Model file for the job. Use its own axes, mm. Face numbers are marked on the shaded views. A direction names the side the tool comes from. Coordinates: 2 decimals unless noted, no trailing zeros. Write each loop counter-clockwise with the first axis right and the second up, starting at its lowest first coordinate (ties: lowest second). Pieces come first, ordered by that corner, then holes. Notation, with made-up numbers: M -22,67 L -3,67 A21 ccw -3,85 Z; hole C 22,7 d4. An arc over 180 degrees is marked long. Put each result on its own line as item: value. Start each with the question number.
Q1. Drop flat-ended pins along their axis: pin 1 (4.5 mm diameter, centred on x = 13.5, y = -1.5, fed in from -Z); pin 2 (0.8 mm diameter, centred on y = -2.5, z = 1.5, fed in from +X). Give the stop position or say it passes through.
Q2. Cut at A-A (x = 17.75). Write the cut outline in (y, z), then the cut area to 3 significant figures.
Q3. Which spindle directions (+Z, -Z, +X, -X, +Y, -Y) get a long thin tool onto all of the face, cutting with end or side? Do the marked faces 1 and 2. Say none if no direction does.
Q4. Cut at C-C (z = 5.75). Write the cut outline in (x, y), then the cut area to 3 significant figures.
Q5. Pull direction X, two halves, no side cores. Call the marked faces 3, 4 and 5: pulls with the +X half, pulls with the -X half, needs draft (parallel to the pull), parting line crosses it, or undercut.
Q6. Cut at D-D (x = 14.25). Write the cut outline in (y, z).
Q7. Cut at B-B (y = 3.25). Write the cut outline in (x, z).
Q8. Drill centre lines: line 1 along Y through (x, z) = (26, 7.5); line 2 along X through (y, z) = (-1.25, 1.25); line 3 along X through (y, z) = (-4.5, 9.75). Where is each one in solid material? Low to high.
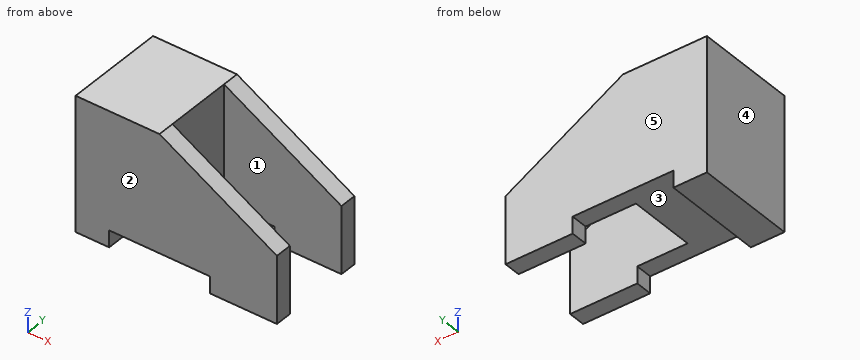
```python
from build123d import *

# Parameters (mm, degrees)
F0_W     = 12.5
F0_H     = 20
F1_DEPTH = 7.5
F3_DEPTH = 2.5
F5_DEPTH = 2.5
F6_W     = 15
F6_H     = 2.5
F7_DEPTH = 15


with BuildPart() as f1:
    # F0 (on Front) → F1 (new body, symmetric)
    with BuildSketch(Plane.XZ):
        with Locations((6.25, 10)):
            Rectangle(F0_W, F0_H)
    extrude(amount=F1_DEPTH, both=True)

    # F2 (on face) → F3 (join)
    with BuildSketch(Plane.XZ.offset(7.5)):
        Polygon((12.5, 20), (12.5, 0), (30, 0), (30, 10), align=None)
    extrude(amount=-F3_DEPTH)

    # F4 (on face) → F5 (join)
    with BuildSketch(Plane(origin=(0, 7.5, 0), x_dir=(-1, 0, 0), z_dir=(0, 1, 0))):
        Polygon((-30, 0), (-12.5, 0), (-12.5, 20), (-30, 10), align=None)
    extrude(amount=-F5_DEPTH)

    # F6 (on face) → F7 (cut, through all)
    with BuildSketch(Plane.XZ.offset(7.5)):
        with Locations((12.5, 1.25)):
            Rectangle(F6_W, F6_H)
    extrude(amount=-F7_DEPTH, mode=Mode.SUBTRACT)


solid = f1.part
```
Computed values:
1. pin 1: z = 2.5
1. pin 2: x = 5
2. outline: M -7.5,2.5 L -5,2.5 L -5,17 L -7.5,17 Z; M 5,2.5 L 7.5,2.5 L 7.5,17 L 5,17 Z
2. area: 72.5 mm2
3. face 1: +Z, -Z, +X
3. face 2: +Z, -Z, +X, -X, -Y
4. outline: M 0,-7.5 L 30,-7.5 L 30,-5 L 12.5,-5 L 12.5,5 L 30,5 L 30,7.5 L 0,7.5 Z
4. area: 275 mm2
5. face 3: undercut
5. face 4: pulls with the -X half
5. face 5: needs draft
6. outline: M -7.5,2.5 L -5,2.5 L -5,19 L -7.5,19 Z; M 5,2.5 L 7.5,2.5 L 7.5,19 L 5,19 Z
7. outline: M 0,0 L 5,0 L 5,2.5 L 12.5,2.5 L 12.5,20 L 0,20 Z
8. line 1: -7.5 to -5, 5 to 7.5
8. line 2: 0 to 5
8. line 3: 0 to 12.5
